Part model, mm, in its own coordinate system. Face numbers are marked on the shaded views. A direction names the side the tool comes from. Coordinates: 2 decimals unless noted, no trailing zeros. Order: outer loops, then holes, each group sorted by start corner. A loop starts at its lowest first (then second) coordinate and runs counter-clockwise, first axis right, second up.
1) Tool access for the marked faces 1, 2, 3 and 4: list every direction of +Z, -Z, +X, -X, +Y, -Y with a clear straight run to the whole face (end or side of a thin tool).
2) Cut at A-A (y = 1.25). List the corners of the cut face in (x, z).
3) Cut at D-D (x = -56). List the corners of the cut face in (y, z), and give its area (3 significant figures).
4) Cut at C-C (z = 16.5). List the corners of the cut face in (x, y) (3 decimals).
5) Pin check, flat tips, straight feed: pin 1 Ø6 at (x, z) = (-57.5, 29) entering from +Y; pin 2 Ø4.5 at (x, z) = (-55, 30) entering from +Y; pin 3 Ø0.7 at (x, y) = (-48.5, 1.5) entering from -Z; pin 4 Ø3 at (x, z) = (-52.82, 31.9) entering from -Y. Stop position of each tip, or through.
6) Cut at B-B (x = -45.25). Give the number of separate pieces and of enclosed holes in the cut face, and give its area (3 significant figures).
7) Wall check: L1, parallel to Z at x = -42.5, y = -5.08; L2, parallel to Z at x = -52.5, y = 2; L3, parallel to Z at x = -47, y = -3.25. Give the ranges that are in metal, low to high.
8) Mould opens along Z. For the marked faces 5, 6 and 7 say: +Z half, -Z half, draft (parallel to the pull), parting line (faces both ways), or undercut.
```python
from build123d import *

# Parameters (mm, degrees)
F0_W      = 25.4
F0_H      = 10.287
F0_R      = 2.54
F1_DEPTH  = 6.35
F2_R      = 1.016
F2_W      = 2.413
F2_H      = 2.2386033088
F3_DEPTH  = 25.4
F5_DEPTH  = 25.4
F6_R      = 1.905
F7_DEPTH  = 12.7
F8_R      = 0.7687670518
F9_DEPTH  = 12.446
F11_DEPTH = 10.287
F12_W     = 8.7730400264
F12_H     = 4.7847703099
F13_DEPTH = 2.3083774


with BuildPart() as f1:
    # F0 (on Front) → F1 (new body)
    with BuildSketch(Plane.XZ):
        with Locations((-48.4233582392, 32.1346397566)):
            Rectangle(F0_W, F0_H)
        with Locations((-52.8246313334, 31.8967439234)):
            Circle(F0_R, mode=Mode.SUBTRACT)
    extrude(amount=F1_DEPTH)

    # F2 (on face) → F3 (cut)
    with BuildSketch(Plane.YZ.offset(-35.7233582392)):
        with Locations((-5.08, 28.8009606302)):
            Circle(F2_R)
        with Locations((-5.08, 35.3567898273)):
            Circle(F2_R)
        with Locations((-5.1435, 31.6693251953)):
            Rectangle(F2_W, F2_H)
    extrude(amount=-F3_DEPTH, mode=Mode.SUBTRACT)

    # F4 (on face) → F5 (cut)
    with BuildSketch(Plane(origin=(0, 0, 26.9911397566), x_dir=(1, 0, 0), z_dir=(0, 0, -1))):
        Polygon((-44.9340231717, 3.81), (-42.169496417, 6.35), (-61.1233582392, 6.35), (-61.1233582392, 3.81), align=None)
    extrude(amount=-F5_DEPTH, mode=Mode.SUBTRACT)

    # F6 (on face) → F7 (join)
    with BuildSketch(Plane(origin=(0, 0, 26.9911397566), x_dir=(1, 0, 0), z_dir=(0, 0, -1))):
        with Locations((-38.7569256127, 3.2096616924)):
            Circle(F6_R)
    extrude(amount=F7_DEPTH)

    # F8 (on face) → F9 (cut)
    with BuildSketch(Plane(origin=(0, 0, 26.9911397566), x_dir=(1, 0, 0), z_dir=(0, 0, -1))):
        with Locations((-38.6601233606, 5.1122006076)):
            Circle(F8_R)
        with Locations((-40.6594645279, 3.3064639445)):
            Circle(F8_R)
        with Locations((-38.8537278648, 1.3071227771)):
            Circle(F8_R)
        with Locations((-36.8543866975, 3.1128594402)):
            Circle(F8_R)
    extrude(amount=F9_DEPTH, mode=Mode.SUBTRACT)

    # F10 (on face) → F11 (join)
    with BuildSketch(Plane.XY.offset(37.2781397566)):
        Polygon((-51.73950345, 0), (-46.5462200276, 0), (-44.7563417256, 2.3083709979), (-53.529381752, 2.3083709979), align=None)
    extrude(amount=-F11_DEPTH)

    # F12 (on face) → F13 (cut)
    with BuildSketch(Plane(origin=(0, 2.3083709979, 0), x_dir=(-1, 0, 0), z_dir=(0, 1, 0))):
        with Locations((49.1428617388, 32.0255719125)):
            Rectangle(F12_W, F12_H)
    extrude(amount=-F13_DEPTH, mode=Mode.SUBTRACT)


solid = f1.part
```
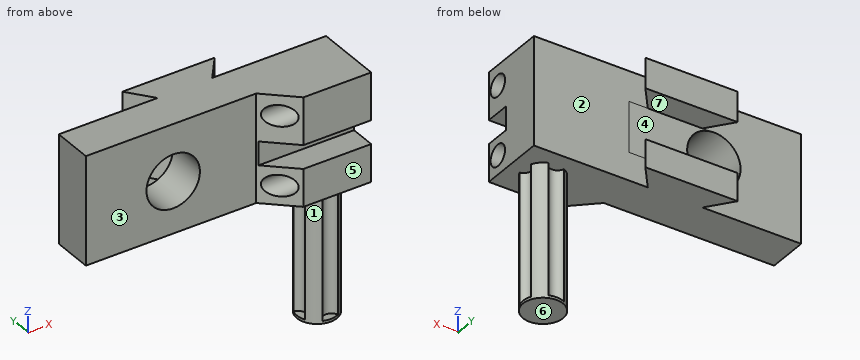
Geometry check:
1. face 1: -Z
1. face 2: +Z, -Z, +X
1. face 3: +Z, -Z, -X, -Y
1. face 4: +X, -X, +Y
2. outline: (-52.71, 26.99) - (-45.58, 26.99) - (-45.58, 29.63) - (-52.71, 29.63) - close; (-52.71, 34.42) - (-45.58, 34.42) - (-45.58, 37.28) - (-52.71, 37.28) - close
3. outline: (-3.81, 26.99) - (0, 26.99) - (0, 37.28) - (-3.81, 37.28) - close
3. area: 39.2 mm2
4. outline: (-40.543, -2.547) arc R0.769 cw to (-40.466, -4.051) arc R1.905 ccw to (-39.42, -4.996) arc R0.769 cw to (-37.916, -4.919) arc R1.905 ccw to (-36.971, -3.873) arc R0.769 cw to (-37.048, -2.369) arc R1.905 ccw to (-38.094, -1.424) arc R0.769 cw to (-39.598, -1.5) arc R1.905 ccw to start
5. pin 1: stops at y = 0
5. pin 2: stops at y = 2.31
5. pin 3: stops at z = 26.99
5. pin 4: passes through
6. separate pieces: 3
6. enclosed holes: 0
6. area: 42.7 mm2
7. L1: z = 26.99 to 27.78, 29.82 to 30.55, 32.79 to 34.34, 36.37 to 37.28
7. L2: z = 26.99 to 29.63, 34.42 to 37.28
7. L3: z = 26.99 to 37.28
8. face 5: draft
8. face 6: -Z half
8. face 7: undercut
